```python
from build123d import *

# Parameters (mm, degrees)
F0_W      = 10
F0_H      = 36
F3_DEPTH  = 3
F2_R      = 6
F4_DEPTH  = 3
F1_R      = 6
F5_DEPTH  = 3
F7_R      = 7.5
F9_DEPTH  = 3
F10_DEPTH = 3
F12_R     = 3.5448933786
F13_DEPTH = 25


with BuildPart() as f3:
    # F0 (on Top) → F3 (new body)
    with BuildSketch(Plane.XY):
        with Locations((5, -18)):
            Rectangle(F0_W, F0_H)
    extrude(amount=F3_DEPTH)

    # F2 (on Top) → F4 (join)
    with BuildSketch(Plane.XY):
        with Locations((5.1598995924, -39.019856602)):
            Circle(F2_R)
    extrude(amount=F4_DEPTH)

    # F1 (on Top) → F5 (join)
    with BuildSketch(Plane.XY):
        with Locations((5.0253178924, 3.6079895217)):
            Circle(F1_R)
    extrude(amount=F5_DEPTH)


with BuildPart() as f9:
    # F7 (on Top) → F9 (new body)
    with BuildSketch(Plane.XY):
        with Locations((-6.096528843, 11.5525964648)):
            Circle(F7_R)
    extrude(amount=F9_DEPTH)


with BuildPart() as f10:
    # F6 (on Top) → F10 (new body)
    with BuildSketch(Plane.XY):
        Polygon((-0.9610534762, 4.1011222638), (2.8653789777, 8.9345108718), (1.0522136364, 10.3699333609), (-2.9573408003, 5.6815163153), align=None)
    extrude(amount=F10_DEPTH)


with BuildPart() as f9_1:
    add(f9.part)

    # F11: union F3, F10
    add(f3.part)
    add(f10.part)

    # F8 (on Top) + F12 (on face) → F13 (cut)
    with BuildSketch(Plane.XY):
        Polygon((-19.6032542735, 13.9494352043), (-6.0890447348, 11.5491952747), (-9.477134794, 23.6695185304), align=None)
    with BuildSketch(Plane(origin=(0, 0, 0), x_dir=(1, 0, 0), z_dir=(0, 0, -1))):
        with Locations((-6.096528843, -11.5525964648)):
            Circle(F12_R)
    extrude(amount=F13_DEPTH, dir=(0, 0, 1), mode=Mode.SUBTRACT)


solid = f9_1.part
```
Model file for the job. Use its own axes, mm. A direction names the side the tool comes from. Coordinates: 2 decimals unless noted, no trailing zeros. Loops run counter-clockwise (first coordinate to the right, second up) from the corner with the lowest first, then second, coordinate; pieces in that order, holes last. Notation, with made-up numbers: (10, -24.75) -> (62, -24.75) arc R12 cw to (62, -3.75) -> close; hole circle Ø5 at (-17.5, 26). An arc over 180 degrees is marked (long way). Answer as a JSON object with one key per item and string values.
Q1. Cut at D-D (x = 9). List the corners of the cut face in (y, z).
Report:
{"outline": "(-43.63, 0) -> (8.1, 0) -> (8.1, 3) -> (-43.63, 3) -> close"}
Q2. Pull direction X, two halves, no side cores. Call faces 1 (the flat face through (4, -13, 0)), 2 (the cylindrical face through (5.27, -45.02, 1.48)), 3 (the flat face through (1.969, 9.644, 1.479)), 4 (the flat face through (10, -18, 1)): released by +X, released by -X, zero draft, split by the parting line, or undercut.
Report:
{"face 1": "zero draft", "face 2": "split by the parting line", "face 3": "undercut", "face 4": "released by +X"}
Q3. Probe probe 1 along X at (y, z) = (-22, 2.15); probe 2 along Y at (x, z) = (-6.75, 1.25); probe 3 along Y at (x, z) = (-3.5, 1.4). List the from-to ranges inside material, lowest first.
Report:
{"probe 1": "x = 0 to 10", "probe 2": "y = 4.08 to 8.07, 15.04 to 19.02", "probe 3": "y = 4.52 to 9.14, 13.97 to 18.59"}
Q4. Cut at C-C (y = -20.5). List the corners of the cut face in (x, z).
Report:
{"outline": "(0, 0) -> (10, 0) -> (10, 3) -> (0, 3) -> close"}
Q5. Cut at B-B (x = -3.75). List the corners of the cut face in (y, z).
Report:
{"outline": "(4.43, 0) -> (8.9, 0) -> (8.9, 3) -> (4.43, 3) -> close; (14.21, 0) -> (18.68, 0) -> (18.68, 3) -> (14.21, 3) -> close"}
Q6. 3-axis set-ups, long thin cutter, end or side, ignore diameter. For faces 5 (the flat face through (0, -18, 1)), 6 (the flat face through (-11.56, 12.52, 1.48)), 7 (the flat face through (-1.612, 4.616, 1.479)): which of +Z, -Z, +X, -X, +Y, -Y reach the whole face in a straight line?
Report:
{"face 5": "+Z, -Z, -X", "face 6": "+Z, -Z, +Y", "face 7": "+Z, -Z, -Y"}
Q7. Flat gauge pins, fed straight in: P1, Ø1.5, axis at y = -25.5, z = 1, coming from the -X side; P2, Ø1, axis at y = 0.5, z = 2.5, coming from the +X side; P3, Ø1.5, axis at x = 7.5, z = 2, coming from the +Y side. Where does each tip first touch, or does it go through?
Report:
{"P1": "stops at x = 0", "P2": "stops at x = 10.43", "P3": "stops at y = 9.35"}
